from build123d import *

# Parameters (mm, degrees)
FASE1_SIZE = 0.35


with BuildPart() as part:
    # Sketch1 → Revolve1 (revolve)
    with BuildSketch(Plane(origin=(0, 0, 0), x_dir=(0, 0, -1), z_dir=(1, 0, 0)), mode=Mode.PRIVATE) as revolve1_sk:
        Polygon((0, 2.5), (2.8, 2.5), (2.8, 1.5), (4, 1.5), (4, 0.5), (2, 0.5), (2, 2), (0, 2), align=None)
    revolve(revolve1_sk.sketch.rotate(Axis((0, 0, 20.700415561), (0, 0, -1)), 90), axis=Axis((0, 0, 20.700415561), (0, 0, -1)))

    # Fase1
    fase1_edges = [part.edges().sort_by_distance(p)[0] for p in [
        (-2.5, 0, -2.8),
    ]]
    chamfer(fase1_edges, length=FASE1_SIZE)


solid = part.part
Source: CAD feature listing. Evaluate the final solid. Frame: model axes, mm. A direction names the side the tool comes from. Give positions to 0.01 mm unless a question says otherwise; leave off trailing zeros. Loops run counter-clockwise (first coordinate to the right, second up) from the corner with the lowest first, then second, coordinate; pieces in that order, holes last. Notation, with made-up numbers: (62.5, 57.25) -> (107.5, 57.25) arc R22 cw to (107.5, 89.25) -> close; hole circle Ø4 at (25.25, 75.5). An arc over 180 degrees is marked (long way). Use a Markdown table: item, result. Add a question column.
1) Section query A-A, the plane y = 0. Return the cut outline in (x, z).
2) Section query C-C, the plane z = -2.3. Return the cut outline in (x, y).
3) Section query D-D, the plane z = -3.3. Return the cut outline in (x, y).
4) Pull-direction query (Y, two-part tool) for faces 3 (the face through (0, 2, -1)), 4 (the face through (-2.5, -0.1, -1.2)), 5 (the face through (1, 0, -4)), 6 (the face through (0.5, -0.5, -2)); classes: +Y half, -Y half, draft (parallel to the pull), parting line (faces both ways), or undercut.
5) First-contact query: pin 1 (1 mm diameter, centred on x = -2, z = -2.5, fed in from +Y); pin 2 (1 mm diameter, centred on y = -1.5, z = -1.5, fed in from +X); pin 3 (2 mm diameter, centred on x = 0, y = 0, fed in from +Z). Flat tips, straight axial feed; report the tip coordinate or a pass-through.
6) Line query: line 1 along Y through (x, z) = (0, -3); line 2 along Y through (x, z) = (0, -1.45); line 3 along Z through (x, y) = (-1.7, 0.75). Output: solid intervals per line, ascending. Write a range as [from, to].
7) Reachability of faces 1 (the face through (-0.108, 0.488, -2.986)), 2 (the face through (0.9, 1.4, -2.8)) from +Z, -Z, +X, -X, +Y, -Y: full face, straight path, thin tool, end or side. Return the list, or none.
Numbers:
| question | item | result |
|---|---|---|
| 1 | outline | (-2.5, -2.45) -> (-2.15, -2.8) -> (-1.5, -2.8) -> (-1.5, -4) -> (-0.5, -4) -> (-0.5, -2) -> (-2, -2) -> (-2, 0) -> (-2.5, 0) -> close; (0.5, -4) -> (1.5, -4) -> (1.5, -2.8) -> (2.15, -2.8) -> (2.5, -2.45) -> (2.5, 0) -> (2, 0) -> (2, -2) -> (0.5, -2) -> close |
| 2 | outline | circle Ø5 at (0, 0); hole circle Ø1 at (0, 0) |
| 3 | outline | circle Ø3 at (0, 0); hole circle Ø1 at (0, 0) |
| 4 | face 3 | undercut |
| 4 | face 4 | parting line |
| 4 | face 5 | draft |
| 4 | face 6 | undercut |
| 5 | pin 1 | stops at y = 2 |
| 5 | pin 2 | stops at x = 2.29 |
| 5 | pin 3 | stops at z = -2 |
| 6 | line 1 | y = [-1.5, -0.5], [0.5, 1.5] |
| 6 | line 2 | y = [-2.5, -2], [2, 2.5] |
| 6 | line 3 | z = [-2.8, -2] |
| 7 | face 1 | +Z, -Z |
| 7 | face 2 | -Z |
